```python
from build123d import *

# Parameters (mm, degrees)
SKETCH1_R           = 7.5
BOSS_EXTRUDE1_DEPTH = 6
SKETCH2_R           = 1.3
CUT_EXTRUDE1_DEPTH  = 84.057209199
LPATTERN1_COUNT     = 4
LPATTERN1_PITCH     = 25
SKETCH3_R           = 3.35
CUT_EXTRUDE2_DEPTH  = 84.057209199


with BuildPart() as part:
    # Sketch1 → Boss-Extrude1 (new body)
    with BuildSketch(Plane.XY):
        with BuildLine():
            Line((75, 7.5), (0, 7.5))
            ThreePointArc((0, 7.5), (5.303300859, 5.303300859), (7.5, 0))
            ThreePointArc((7.5, 0), (5.303300859, -5.303300859), (0, -7.5))
            Line((0, -7.5), (75, -7.5))
            ThreePointArc((75, -7.5), (67.5, 0), (75, 7.5))
        make_face()
        with Locations((75, 0)):
            Circle(SKETCH1_R)
        Circle(SKETCH1_R)
    extrude(amount=BOSS_EXTRUDE1_DEPTH)

    # Sketch2 → Cut-Extrude1 (cut, through all)
    with BuildSketch(Plane.XY.offset(6)):
        Circle(SKETCH2_R)
        with Locations((75, 0)):
            Circle(SKETCH2_R)
    cut_extrude1 = extrude(amount=-CUT_EXTRUDE1_DEPTH, mode=Mode.SUBTRACT)

    # LPattern1: Cut-Extrude1 ×4
    with Locations(*[(i * LPATTERN1_PITCH, 0, 0) for i in range(1, LPATTERN1_COUNT)]):
        add(cut_extrude1, mode=Mode.SUBTRACT)

    # Sketch3 → Cut-Extrude2 (cut, through all)
    with BuildSketch(Plane.XY.offset(6)):
        with Locations((75, 0)):
            Circle(SKETCH3_R)
    extrude(amount=-CUT_EXTRUDE2_DEPTH, mode=Mode.SUBTRACT)


solid = part.part
```
For this review, take the finished solid that the model builds, in its own axes (mm). Coordinates: 2 decimals unless noted, no trailing zeros. Write each loop counter-clockwise with the first axis right and the second up, starting at its lowest first coordinate (ties: lowest second). Pieces come first, ordered by that corner, then holes. Notation, with made-up numbers: (-3.75, 30) - (14.25, 30) arc R22 ccw to (14.25, 45) - close; hole circle Ø3 at (-36, 29.5). An arc over 180 degrees is marked (long way). Put each result on its own line as item: value.
1. Add section C-C, the plane y = 0. Give the boundary of the cut face in (x, z).
Values found:
outline: (-7.5, 0) - (-1.3, 0) - (-1.3, 6) - (-7.5, 6) - close; (1.3, 0) - (23.7, 0) - (23.7, 6) - (1.3, 6) - close; (26.3, 0) - (48.7, 0) - (48.7, 6) - (26.3, 6) - close; (51.3, 0) - (71.65, 0) - (71.65, 6) - (51.3, 6) - close; (78.35, 0) - (82.5, 0) - (82.5, 6) - (78.35, 6) - close
2. Add section B-B, the plane z = 3.1. Give the boundary of the cut face in (x, y), then the cut area to 3 significant figures.
Values found:
outline: (0, -7.5) - (75, -7.5) arc R7.5 ccw to (75, 7.5) - (0, 7.5) arc R7.5 ccw to start; hole circle Ø2.6 at (0, 0); hole circle Ø2.6 at (25, 0); hole circle Ø2.6 at (50, 0); hole circle Ø6.7 at (75, 0)
area: 1,250 mm²
3. Add section D-D, the plane y = 6. Give the boundary of the cut face in (x, z), then the cut area to 3 significant figures.
Values found:
outline: (-4.5, 0) - (79.5, 0) - (79.5, 6) - (-4.5, 6) - close
area: 504 mm²
4. Add section A-A, the plane x = 25. Give the boundary of the cut face in (y, z).
Values found:
outline: (-7.5, 0) - (-1.3, 0) - (-1.3, 6) - (-7.5, 6) - close; (1.3, 0) - (7.5, 0) - (7.5, 6) - (1.3, 6) - close
5. Wall thickness on probe 1 along X at (y, z) = (-0.5, 1.95); probe 2 along Y at (x, z) = (50, 1.35); probe 3 along Y at (x, z) = (1, 0.45): over which ranges is each line inside the solid? List them lowest first.
Values found:
probe 1: -7.48 to -1.2, 1.2 to 23.8, 26.2 to 48.8, 51.2 to 71.69, 78.31 to 82.48
probe 2: -7.5 to -1.3, 1.3 to 7.5
probe 3: -7.5 to -0.83, 0.83 to 7.5
6. Mouldability with a two-part tool opening along Y and no side actions: class faces 1 (the cylindrical face through (48.7, 0.06, 3.04)), 2 (the cylindrical face through (-0.17, 1.29, 3.04)), 3 (the flat face through (37, -7.5, 3)), 4 (the flat face through (38, 7.5, 3)) as released by +Y, released by -Y, zero draft, split by the parting line, or undercut.
Values found:
face 1: undercut
face 2: undercut
face 3: released by -Y
face 4: released by +Y
